Autodesk Inventor part; units mm, degrees
ref_plane "YZ Plane" through (0, 0, 0) normal (1, 0, 0) x (0, 1, 0)
ref_plane "XZ Plane" through (0, 0, 0) normal (0, 1, 0) x (-1, 0, 0)
ref_plane "XY Plane" through (0, 0, 0) normal (0, 0, 1) x (1, 0, 0)
sketch "Sketch1" plane through (0, 0, 0) normal (0, 0, 1) x (1, 0, 0)
  line L0 (0, 67.3) -> (0, 0)
  line L1 (0, 0) -> (60, 0)
  line L2 (60, 0) -> (60, 16)
  line L3 (60, 16) -> (8, 67.3)
  line L4 (8, 67.3) -> (0, 67.3)
  dimension "d0" = 67.3
  dimension "d1" = 8
  dimension "d2" = 16
  dimension "d3" = 60
extrude "Extrusion1" add sketch "Sketch1" along normal blind 6
sketch "Sketch2" plane through (0, 0, 6) normal (0, 0, 1) x (1, 0, 0)
  line L0 (0, 67.3) -> (0, 0)
  line L1 (0, 0) -> (60, 0)
  line L2 (60, 0) -> (60, 16)
  line L3 (8, 67.3) -> (0, 67.3)
  line L4 (16.3, 50.05) -> (16.3, 45.55)
  line L5 (0, 45.55) -> (0, 50.05)
  line L6 (5, 52.55) -> (12.3, 52.55)
  line L7 (12.3, 43.05) -> (5, 43.05)
  line L8 (38.25, 16.3) -> (42.75, 16.3)
  line L9 (42.75, 0) -> (38.25, 0)
  line L10 (45.25, 12.3) -> (45.25, 5)
  line L11 (35.75, 5) -> (35.75, 12.3)
  line L12 (5, 43.05) -> (5, 45.55)
  line L13 (5, 50.05) -> (5, 52.55)
  line L14 (12.3, 52.55) -> (12.3, 50.05)
  line L15 (12.3, 45.55) -> (12.3, 43.05)
  line L16 (0, 50.05) -> (5, 50.05)
  line L17 (12.3, 50.05) -> (16.3, 50.05)
  line L18 (16.3, 45.55) -> (12.3, 45.55)
  line L19 (5, 45.55) -> (0, 45.55)
  line L20 (35.75, 12.3) -> (38.25, 12.3)
  line L21 (42.75, 12.3) -> (45.25, 12.3)
  line L22 (45.25, 5) -> (42.75, 5)
  line L23 (38.25, 5) -> (35.75, 5)
  line L24 (38.25, 0) -> (38.25, 5)
  line L25 (38.25, 12.3) -> (38.25, 16.3)
  line L26 (42.75, 16.3) -> (42.75, 12.3)
  line L27 (42.75, 5) -> (42.75, 0)
  point P0 (16.3, 47.8)
  point P1 (40.5, 16.3)
  dimension "d6" = 4.5
  dimension "d7" = 5
  dimension "d8" = 7.3
  dimension "d9" = 4
  dimension "d10" = 2.5
  dimension "d11" = 19.5
  dimension "d12" = 19.5
extrude "Extrusion2" cut sketch "Sketch2" against normal blind 6
sketch "Sketch3" plane through (0, 0, 6) normal (0, 0, 1) x (1, 0, 0)
  line L0 (0, 45.55) -> (0, 0)
  line L1 (0, 0) -> (38.25, 0)
  line L2 (38.25, 16.3) -> (42.75, 16.3)
  line L3 (42.75, 0) -> (60, 0)
  line L4 (0, 67.3) -> (0, 50.05)
  line L5 (16.3, 50.05) -> (16.3, 45.55)
  line L6 (0, 40.3) -> (-4, 40.3)
  line L7 (-6, 38.3) -> (-6, 34.3)
  line L8 (-4, 32.3) -> (0, 32.3)
  line L9 (0, 32.3) -> (0, 40.3)
  line L10 (0, 63.3) -> (-4, 63.3)
  line L11 (-6, 61.3) -> (-6, 57.3)
  line L12 (-4, 55.3) -> (0, 55.3)
  line L13 (0, 55.3) -> (0, 63.3)
  line L14 (25, 0) -> (33, 0)
  line L15 (33, 0) -> (33, -4)
  line L16 (31, -6) -> (27, -6)
  line L17 (25, -4) -> (25, 0)
  line L18 (48, 0) -> (56, 0)
  line L19 (56, 0) -> (56, -4)
  line L20 (54, -6) -> (50, -6)
  line L21 (48, -4) -> (48, 0)
  arc A0 (-4, 63.3) -> (-6, 61.3) centre (-4, 61.3) ccw
  arc A1 (-6, 57.3) -> (-4, 55.3) centre (-4, 57.3) ccw
  arc A2 (-4, 40.3) -> (-6, 38.3) centre (-4, 38.3) ccw
  arc A3 (-6, 34.3) -> (-4, 32.3) centre (-4, 34.3) ccw
  arc A4 (25, -4) -> (27, -6) centre (27, -4) ccw
  arc A5 (31, -6) -> (33, -4) centre (31, -4) ccw
  arc A6 (48, -4) -> (50, -6) centre (50, -4) ccw
  arc A7 (54, -6) -> (56, -4) centre (54, -4) ccw
  point P0 (16.3, 47.8)
  point P1 (40.5, 16.3)
  dimension "d15" = 2
  dimension "d16" = 8
  dimension "d17" = 8
  dimension "d18" = 8
  dimension "d19" = 8
  dimension "d20" = 6
  dimension "d21" = 6
  dimension "d22" = 15
  dimension "d23" = 15
  dimension "d24" = 7.5
  dimension "d25" = 7.5
extrude "Extrusion3" add sketch "Sketch3" against normal blind 6
properties part number "y_motor_mount_brace"
The listing builds one solid part. Answer for the finished solid, in the listing's coordinates (mm). A direction names the side the tool comes from. Give positions to 0.01 mm unless a question says otherwise; leave off trailing zeros. Order: outer loops, then holes, each group sorted by start corner. A loop starts at its lowest first (then second) coordinate and runs counter-clockwise, first axis right, second up.
1) Determine the mould class of faces 1 (the face through (0, 43, 3)), 2 (the face through (-2, 63.3, 3)), 3 (the face through (38.25, 14, 3)) for opening direction X: pulls with the +X half, pulls with the -X half, needs draft (parallel to the pull), parting line crosses it, or undercut.
Reported:
face 1: pulls with the -X half
face 2: needs draft
face 3: undercut
2) Find section A-A on y = 11. Write down the section's boundary in (x, z), then the cut area to 3 significant figures.
Reported:
outline: (0, 0) - (35.75, 0) - (35.75, 6) - (0, 6) - close; (45.25, 0) - (60, 0) - (60, 6) - (45.25, 6) - close
area: 303 mm2
3) Given P1, Ø3, axis at y = -2, z = 2.5, coming from the -X side; P2, Ø3, axis at x = 44, z = 2.5, coming from the -Y side; P3, Ø1.5, axis at y = 1.5, z = 2.5, coming from the -X side, each flat-ended and moving along its own axis, determine where each tip first touches the part or whether it passes through.
Reported:
P1: stops at x = 25
P2: stops at y = 0
P3: stops at x = 0
4) Find section C-C on y = 30. Write down the section's boundary in (x, z).
Reported:
outline: (0, 0) - (45.81, 0) - (45.81, 6) - (0, 6) - close
5) Find section B-B on x = 2.5. Write down the section's boundary in (y, z).
Reported:
outline: (0, 0) - (45.55, 0) - (45.55, 6) - (0, 6) - close; (50.05, 0) - (67.3, 0) - (67.3, 6) - (50.05, 6) - close
6) For faces 4 (the face through (5, 51, 3)), 5 (the face through (42.75, 3, 3)), 6 (the face through (0, 16, 3)), determine the directions among +Z, -Z, +X, -X, +Y, -Y from which every point of the face is accessible in a straight line to the end or side of a thin tool.
Reported:
face 4: +Z, -Z
face 5: +Z, -Z, -Y
face 6: +Z, -Z, -X, -Y
7) Consider line 1 along X through (y, z) = (2, 4.55); line 2 along Y through (x, z) = (6, 5.75); line 3 along Y through (x, z) = (4.5, 3.3). Determine where each line is inside the solid, lowest interval first.
Reported:
line 1: x = 0 to 38.25, 42.75 to 60
line 2: y = 0 to 43.05, 52.55 to 67.3
line 3: y = 0 to 45.55, 50.05 to 67.3
8) Find section D-D on x = 51. Write down the section's boundary in (y, z), then the cut area to 3 significant figures.
Reported:
outline: (-6, 0) - (24.88, 0) - (24.88, 6) - (-6, 6) - close
area: 185 mm2
